Geometry: final body of the model. Coordinates: model frame, mm. A direction names the side the tool comes from. Give positions to 0.01 mm unless a question says otherwise; leave off trailing zeros. Loops run counter-clockwise (first coordinate to the right, second up) from the corner with the lowest first, then second, coordinate; pieces in that order, holes last.
Autodesk Inventor part; units mm, degrees
ref_plane "Work Plane1" through (5.2813, 23, 0) normal (0, 1, 0) x (1, 0, 0)
ref_plane "Work Plane2" through (52.4294, 18.8912, 0) normal (0.678674, 0.7344396, 0) x (-0.7344396, 0.678674, 0)
ref_plane "YZ Plane" through (0, 0, 0) normal (1, 0, 0) x (0, 1, 0)
sketch "Sketch1" plane through (0, 0, 0) normal (0, 0, 1) x (1, 0, 0)
  line L0 (0, 0) -> (39.2539, 0)
  line L1 (40, 13) -> (0, 13)
  line L2 (0, 13) -> (0, 0)
  circle A0 centre (4, 6.5) radius 4
  circle A1 centre (4, 6.5) radius 2.5
  line L3 (8, 13) -> (8, 0)
  arc A2 (5.2813, 13) -> (1.7572, 2) centre (6.6406, 6.5) ccw
  line L4 (40, 0) -> (55, 0)
  line L5 (55, 0) -> (55, 13)
  arc A3 (47.5, 21) -> (40, 13) centre (49.851, 11.2803) ccw
  line L6 (54.25, 12.35) -> (40.5638, 0.4886)
  arc A4 (54.9201, 14.1433) -> (47.5, 21) centre (47, 13.0156) ccw
  arc A5 (39.2539, 0) -> (40.5638, 0.4886) centre (39.2539, 2) ccw
  arc A6 (54.25, 12.35) -> (54.9201, 14.1433) centre (52.9401, 13.8614) ccw
  line L7 (8, 0) -> (8, 2)
  line L8 (8, 2) -> (-2, 2)
  line L9 (-2, 2) -> (-2, 0)
  line L10 (-2, 0) -> (8, 0)
  point P0 (0, 6.5)
  point P1 (0, 2)
  dimension "d2" = 8
  dimension "d0" = 40
  dimension "d3" = 5
  dimension "d4" = 15
  dimension "d5" = 13
  dimension "d7" = 10
  dimension "d8" = 8
  dimension "d9" = 2
  dimension "d10" = 2
  dimension "d11" = 10
extrude "Extrusion1" add sketch "Sketch1" along normal blind 15 contours L2 L8 L3 L0 | L3 L1 A3 A4 A6 L6 A5 L0 | L8 A2 A0 L3 | A2 L1 L3 A0 | A0
ref_plane "Work Plane1" through (5.2813, 23, 0) normal (0, 1, 0) x (1, 0, 0)
sketch "Sketch2" plane through (5.2813, 23, 0) normal (0, 1, 0) x (1, 0, 0)
  line L0 (-5.2813, 0) -> (-5.2813, -15)
  line L1 (-5.2813, -7.5) -> (-5.2813, -5)
  line L2 (-5.2813, -7.5) -> (-5.2813, -10)
  line L3 (-5.2813, -5) -> (9.7187, -5)
  line L4 (-5.2813, -10) -> (9.7187, -10)
  line L5 (9.7187, -10) -> (9.7187, -5)
  line L6 (9.7187, -7.5) -> (9.7187, -6)
  line L7 (9.7187, -7.5) -> (9.7187, -9)
  line L8 (9.7187, -9) -> (24.7188, -9)
  line L9 (24.7188, -9) -> (24.7188, -6)
  line L10 (24.7188, -6) -> (9.7187, -6)
  dimension "d15" = 2.5
  dimension "d16" = 2.5
  dimension "d17" = 15
  dimension "d18" = 15
  dimension "d19" = 1.5
  dimension "d20" = 1.5
  dimension "d21" = 15
extrude "Extrusion2" cut sketch "Sketch2" against normal through all contours L3 L5 L4 L0
sketch "Sketch3" plane through (15, 0, 5) normal (-1, 0, 0) x (0, 0, 1)
  line L0 (0, 13) -> (5, 13)
  circle A0 centre (2.5, 11) radius 1.5
  circle A1 centre (2.5, 2) radius 1.5
  line L1 (5, 0) -> (0, 0)
  point P0 (-5, 0)
  point P1 (2.5, 0)
  dimension "d25" = 3
  dimension "d27" = 3
extrude "Extrusion3" cut sketch "Sketch3" against normal through all contours A1
extrude "Extrusion4" cut sketch "Sketch3" against normal blind 26 contours A0
extrude "Extrusion5" cut sketch "Sketch2" against normal blind 12 contours L10 L9 L8 L5
ref_plane "Work Plane2" through (52.4294, 18.8912, 0) normal (0.678674, 0.7344396, 0) x (-0.7344396, 0.678674, 0)
sketch "Sketch4" plane through (52.4294, 18.8912, 0) normal (0.678674, 0.7344396, 0) x (-0.7344396, 0.678674, 0)
  circle A0 centre (0, 7.5) radius 1.5
  point P0 (25.6853, 0)
  point P1 (5.0516, 15)
  point P2 (-5.0516, 15)
  dimension "d34" = 3
loft "Loft1" cut profiles "Sketch4" section 2 edges at (41, 11, 6)
properties part number "ProjEnAble_Finger"
Q1. Material intervals for probe 1 along Z at (x, y) = (36.25, 2); probe 2 along Z at (x, y) = (6.5, 9.5); probe 3 along X at (y, z) = (6.5, 11.4), sorted ascending.
Q2. Section query C-C, the plane x = 34. Return loops of the section in (y, z).
Q3. Reachability of faces 4 (the face through (22.9, 13, 5.7)), 5 (the face through (22, 12, 9)), 6 (the face through (7, 7, 10)) from +Z, -Z, +X, -X, +Y, -Y: full face, straight path, thin tool, end or side. Return the list, or none.
Q4. Section query B-B, the plane z = 11.25. Return loops of the section in (x, y), and give its area (3 significant figures).
Q5. Section query D-D, the plane y = 8.5. Return loops of the section in (x, z).
Q6. Pin query (flat end, axial travel): pin 1 Ø5 at (y, z) = (2, 7.5) entering from +X; pin 2 Ø0.9 at (x, z) = (0.5, 12.5) entering from +Y; pin 3 Ø1.5 at (y, z) = (14.5, 3) entering from -X. Return the tip coordinate at first contact, or that it passes through.
Q7. Section query A-A, the plane x = 17. Return loops of the section in (y, z), and give its area (3 significant figures).
Q8. Mould query, pull axis Z, two halves, no side actions, for faces 1 (the face through (47.5, 6.5, 7.4)), 2 (the face through (27, 8, 0)), 3 (the face through (7, 7, 5)). Classes: +Z half, -Z half, draft (parallel to the pull), parting line (faces both ways), or undercut.
Resolved:
1. probe 1: z = 0 to 6, 9 to 15
1. probe 2: z = 0 to 5, 10 to 15
1. probe 3: x = 0 to 1.5, 6.5 to 47.5
2. outline: (0, 0) - (13, 0) - (13, 15) - (0, 15) - close; hole circle Ø3 at (2, 7.5); hole circle Ø3 at (11, 7.5)
3. face 4: +Z, -Z, -X, +Y
3. face 5: -X, +Y
3. face 6: -X, +Y, -Y
4. outline: (0, 0) - (39.25, 0) arc R2 ccw to (40.56, 0.49) - (54.25, 12.35) arc R2 ccw to (54.92, 14.14) arc R8 ccw to (47.5, 21) arc R10 ccw to (40, 13) - (5.28, 13) arc R6.64 ccw to (1.76, 2) - (0, 2) - close; hole circle Ø5 at (4, 6.5)
4. area: 675 mm2
5. outline: (0.31, 0) - (2.5, 0) - (2.5, 5) - (0.31, 5) - close; (0.31, 10) - (2.5, 10) - (2.5, 15) - (0.31, 15) - close; (5.5, 0) - (49.81, 0) - (49.81, 15) - (5.5, 15) - (5.5, 10) - (15, 10) - (15, 5) - (5.5, 5) - close
6. pin 1: stops at x = 45.19
6. pin 2: stops at y = 9.92
6. pin 3: stops at x = 40.16
7. outline: (0, 0) - (13, 0) - (13, 6) - (11, 6) arc R1.5 cw to (11, 9) - (13, 9) - (13, 15) - (0, 15) - close; hole circle Ø3 at (2, 7.5)
7. area: 178 mm2
8. face 1: draft
8. face 2: -Z half
8. face 3: undercut
